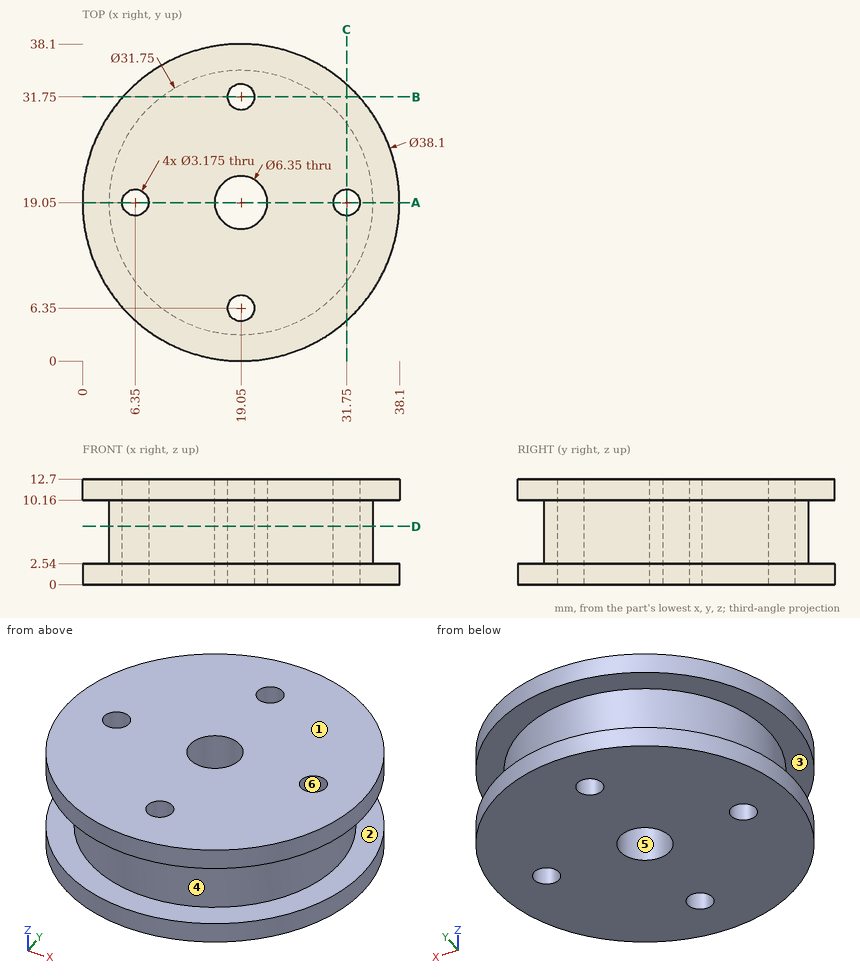
Check sheet for the drawn part. Datum: minimum x, y, z corner. Units: mm. A direction names the side the tool comes from. Round coordinates to 2 decimals unless told otherwise and drop trailing zeros. Loops run counter-clockwise (first coordinate to the right, second up) from the corner with the lowest first, then second, coordinate; pieces in that order, holes last. Notation, with made-up numbers: (5, 72.5) - (53, 72.5) arc R36 cw to (53, 110.5) - close; hole circle Ø9 at (61.25, 13.5). An arc over 180 degrees is marked (long way). Answer as a JSON object with one key per item and string values. Group by question number.
Q1. Sectioned sample at B-B, the plane y = 31.75. Enter the section's corners in (x, z) (1 decimal), plus the area to 3 significant figures.
Q2. Scan lines: line 1 along Y through (x, z) = (19.05, 7) (1 decimal); line 2 along Z through (x, y) = (30.5, 31); line 3 along X through (y, z) = (18.5, 12.25). Record each from-to range of solid material in increasing order. Write a range as [from, to].
Q3. Set-up check for the marked faces 1 and 2: record each of +Z, -Z, +X, -X, +Y, -Y from which the full face is reachable in a straight line by a thin tool's end or side.
Q4. Mould release check, pull along Y, two halves, no side actions. Record for the marked faces 3, 4, 5 and 6: released by +Y, released by -Y, zero draft, split by the parting line, or undercut.
Q5. Sectioned sample at D-D, the plane z = 7. Count the separate pieces of the cut face and the enclosed holes in it, plus the area to 3 significant figures.
Q6. Gauge pin test, flat ends, axial feed: P1, Ø3, axis at y = 22.5, z = 10, coming from the -X side; P2, Ø1.5, axis at x = 7, z = 8.5, coming from the -Y side; P3, Ø4, axis at y = 30, z = 6, coming from the -X side. Record the tip position at first contact, or that the pin passes through.
Q7. Sectioned sample at A-A, the plane y = 19.05. Enter the section's corners in (x, z) (1 decimal).
Solution:
{
 "1": {"outline": "(4.9, 0) - (17.5, 0) - (17.5, 12.7) - (4.9, 12.7) - (4.9, 10.2) - (9.5, 10.2) - (9.5, 2.5) - (4.9, 2.5) - close; (20.6, 0) - (33.2, 0) - (33.2, 2.5) - (28.6, 2.5) - (28.6, 10.2) - (33.2, 10.2) - (33.2, 12.7) - (20.6, 12.7) - close", "area": "249 mm²"},
 "2": {"line 1": "y = [3.2, 4.8], [7.9, 15.9], [22.2, 30.2], [33.3, 34.9]", "line 2": "z = [0, 2.54], [10.16, 12.7]", "line 3": "x = [0.01, 4.86], [7.84, 15.92], [22.18, 30.26], [33.24, 38.09]"},
 "3": {"face 1": "+Z, +X, -X, +Y, -Y", "face 2": "none"},
 "4": {"face 3": "zero draft", "face 4": "split by the parting line", "face 5": "undercut", "face 6": "undercut"},
 "5": {"separate pieces": "1", "enclosed holes": "5", "area": "728 mm²"},
 "6": {"P1": "stops at x = 0.1", "P2": "stops at y = 7.9", "P3": "stops at x = 5.94"},
 "7": {"outline": "(0, 0) - (4.8, 0) - (4.8, 12.7) - (0, 12.7) - (0, 10.2) - (3.2, 10.2) - (3.2, 2.5) - (0, 2.5) - close; (7.9, 0) - (15.9, 0) - (15.9, 12.7) - (7.9, 12.7) - close; (22.2, 0) - (30.2, 0) - (30.2, 12.7) - (22.2, 12.7) - close; (33.3, 0) - (38.1, 0) - (38.1, 2.5) - (34.9, 2.5) - (34.9, 10.2) - (38.1, 10.2) - (38.1, 12.7) - (33.3, 12.7) - close"}
}
